Geometry: see drawing. Coordinates: mm, zero at the bounding-box minimum. Round coordinates to 2 decimals unless told otherwise and drop trailing zeros. Order: outer loops, then holes, each group sorted by start corner. A loop starts at its lowest first (then second) coordinate and runs counter-clockwise, first axis right, second up. Notation, with made-up numbers: (4.25, 0) -> (30.25, 0) arc R11 cw to (30.25, 20) -> close; hole circle Ø11 at (-2.5, -3). An arc over 180 degrees is marked (long way). Answer as CSV lines item,"result". Start each with the question number.
(1) Section query A-A (z = 31). Output: boundary loops of the cut face in (x, y), plus the area to 3 significant figures.
(2) Section query B-B (y = 4.25). Output: boundary loops of the cut face in (x, z), plus the area to 3 significant figures.
(3) Contact query for a flat-ended pin moving along its axis: P1, Ø9.5, axis at x = 215.5, y = 10, coming from the -Z side. Output: stop coordinate, or through.
(4) Line query: line 1 along X through (y, z) = (7.25, 11); line 2 along Z through (x, y) = (212, 14.75). Output: solid intervals per line, ascending. Write a range as from..to.
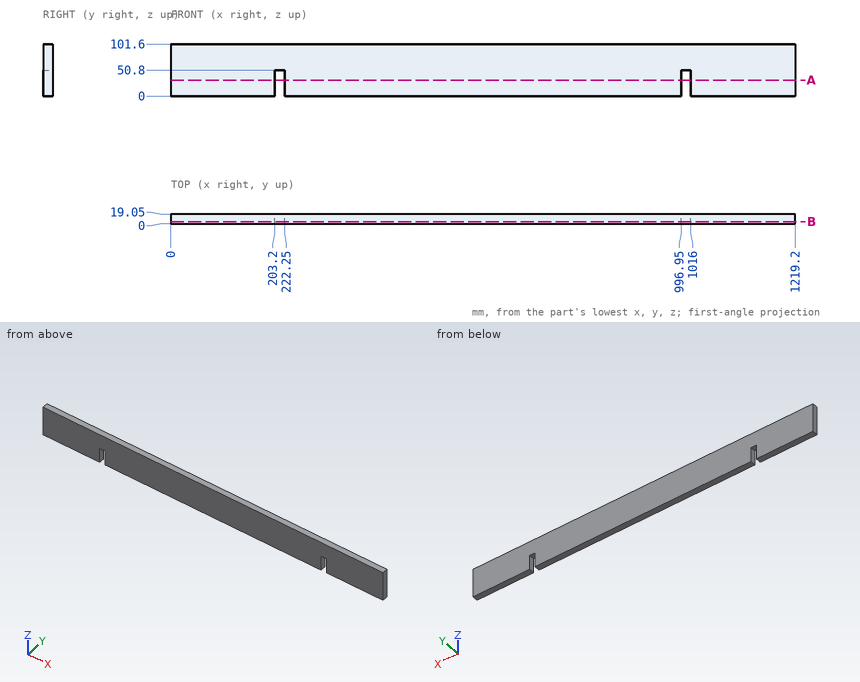
Answer block:
1,outline,"(0, 0) -> (203.2, 0) -> (203.2, 19.05) -> (0, 19.05) -> close; (222.25, 0) -> (996.95, 0) -> (996.95, 19.05) -> (222.25, 19.05) -> close; (1016, 0) -> (1219.2, 0) -> (1219.2, 19.05) -> (1016, 19.05) -> close"
1,area,"22,500 mm2"
2,outline,"(0, 0) -> (203.2, 0) -> (203.2, 50.8) -> (222.25, 50.8) -> (222.25, 0) -> (996.95, 0) -> (996.95, 50.8) -> (1016, 50.8) -> (1016, 0) -> (1219.2, 0) -> (1219.2, 101.6) -> (0, 101.6) -> close"
2,area,"122,000 mm2"
3,P1,"z = 50.8"
4,line 1,"0..203.2, 222.25..996.95, 1016..1219.2"
4,line 2,"50.8..101.6"
